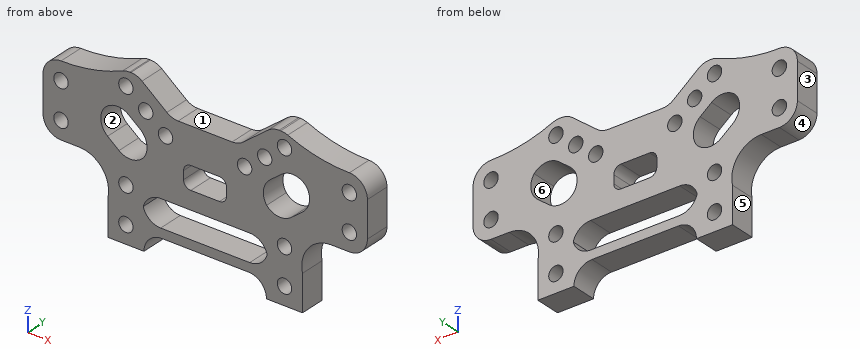
```python
from build123d import *

# Parameters (mm, degrees)
F0_R        = 1
F1_DEPTH    = 3.5
F2_R        = 2.49999
F3_W        = 8.6775156483
F3_H        = 3.7365088891
F4_DEPTH    = 25.4
F5_T1_DEPTH = 3.5
F6_W        = 5.9684215951
F6_H        = 3.1480632909
F7_DEPTH    = 25.4
F8_R        = 1


# Not quite as in the source:
# - a fillet or chamfer that OpenCascade refuses, or shapes differently, is made with other operations: its cross-section is extruded or revolved along the edge and cut away or added
# - a fillet or chamfer is up to 0.001 mm smaller than in the source, because OpenCascade refuses the exact size


with BuildPart() as f1:
    # F0 (on Front) → F1 (new body)
    with BuildSketch(Plane.XZ):
        with BuildLine():
            Line((-13.8224843517, 17.5), (-13.8224843517, 10))
            Line((-13.8224843517, 10), (-13.8224843517, 7.5))
            Line((-13.8224843517, 7.5), (-8.8224843517, 7.5))
            ThreePointArc((-8.8224843517, 7.5), (-5.620922233, 5.961249695), (-4.8224843517, 2.5))
            Line((-4.8224843517, 2.5), (-4.8224843517, 0))
            Line((-4.8224843517, 0), (-4.8224843517, -2.5))
            Line((-4.8224843517, -2.5), (0.1775156483, -2.5))
            Line((0.1775156483, -2.5), (0.1775156483, 0))
            Line((0.1775156483, 0), (8.6775156483, 0))
            Line((8.6775156483, 0), (17.1775156483, 0))
            Line((17.1775156483, 0), (17.1775156483, -2.5))
            Line((17.1775156483, -2.5), (22.1775156483, -2.5))
            Line((22.1775156483, -2.5), (22.1775156483, 0))
            Line((22.1775156483, 0), (22.1775156483, 2.5))
            ThreePointArc((22.1775156483, 2.5), (22.9759535296, 5.961249695), (26.1775156483, 7.5))
            Line((26.1775156483, 7.5), (31.1775156483, 7.5))
            Line((31.1775156483, 7.5), (31.1775156483, 10))
            Line((31.1775156483, 10), (31.1775156483, 17.5))
            Line((31.1775156483, 17.5), (28.6775156483, 17.5))
            ThreePointArc((28.6775156483, 17.5), (24.0740626287, 17.9907408644), (19.6775156483, 19.4409066995))
            Line((19.6775156483, 19.4409066995), (18.069904763, 19.4409066995))
            Line((18.069904763, 19.4409066995), (13.2764897522, 15.6480632909))
            Line((13.2764897522, 15.6480632909), (4.0469631395, 15.6480632909))
            Line((4.0469631395, 15.6480632909), (-0.7712156733, 19.4605013357))
            Line((-0.7712156733, 19.4605013357), (-2.3224843517, 19.4605013357))
            ThreePointArc((-2.3224843517, 19.4605013357), (-6.7169560029, 17.9958056322), (-11.3224843517, 17.5))
            Line((-11.3224843517, 17.5), (-13.8224843517, 17.5))
        make_face()
        with Locations((-2.3224843517, 0)):
            Circle(F0_R, mode=Mode.SUBTRACT)
        with Locations((-2.3224843517, 5)):
            Circle(F0_R, mode=Mode.SUBTRACT)
        with BuildLine():
            ThreePointArc((18.6775156483, 0), (19.6775156483, 1), (20.6775156483, 0))
            ThreePointArc((20.6775156483, 0), (19.6775156483, -1), (18.6775156483, 0))
        make_face(mode=Mode.SUBTRACT)
        with Locations((19.6775156483, 5)):
            Circle(F0_R, mode=Mode.SUBTRACT)
        with BuildLine():
            ThreePointArc((-12.3224843517, 10), (-11.3224843517, 11), (-10.3224843517, 10))
            ThreePointArc((-10.3224843517, 10), (-11.3224843517, 9), (-12.3224843517, 10))
        make_face(mode=Mode.SUBTRACT)
        with Locations((3.1775156483, 13.1480632909)):
            Circle(F0_R, mode=Mode.SUBTRACT)
        with Locations((-11.3224843517, 15)):
            Circle(F0_R, mode=Mode.SUBTRACT)
        with Locations((0.4275156483, 15.3240316454)):
            Circle(F0_R, mode=Mode.SUBTRACT)
        with Locations((-2.3224843517, 17.5)):
            Circle(F0_R, mode=Mode.SUBTRACT)
        with Locations((14.1459372434, 13.1480632909)):
            Circle(F0_R, mode=Mode.SUBTRACT)
        with Locations((28.6775156483, 10)):
            Circle(F0_R, mode=Mode.SUBTRACT)
        with Locations((16.9275156483, 15.3240316454)):
            Circle(F0_R, mode=Mode.SUBTRACT)
        with Locations((19.6775156483, 17.5)):
            Circle(F0_R, mode=Mode.SUBTRACT)
        with Locations((28.6775156483, 15)):
            Circle(F0_R, mode=Mode.SUBTRACT)
    extrude(amount=F1_DEPTH)

    # F2 (radius 2.5 in the source; OpenCascade refuses exactly that, so slightly less here)
    f2_edges = [f1.edges().sort_by_distance(p)[0] for p in [
        (-13.822484, -1.75, 17.5),
        (-13.822484, -1.75, 7.5),
        (31.177516, -1.75, 7.5),
        (31.177516, -1.75, 17.5),
        (-2.322484, -1.75, 19.460501),
        (-0.771216, -1.75, 19.460501),
        (4.046963, -1.75, 15.648063),
        (13.27649, -1.75, 15.648063),
        (18.069905, -1.75, 19.440907),
        (19.677516, -1.75, 19.440907),
        (0.177516, -1.75, 0),
        (17.177516, -1.75, 0),
    ]]
    fillet(f2_edges, radius=F2_R)

    # F3 (on face) → F4 (cut)
    with BuildSketch(Plane.XZ.offset(3.5)):
        Polygon((1.6262469699, 11.1875619551), (-3.8737530301, 15.5394986643), (-6.8168965969, 11.8199386845), (-1.3168965969, 7.4680019754), align=None)
        with Locations((4.3387578242, 3.1317455554)):
            Rectangle(F3_W, F3_H)
        with Locations((13.0162734725, 3.1317455554)):
            Rectangle(F3_W, F3_H)
        Polygon((24.1719278936, 11.8199386845), (21.2287843267, 15.5394986643), (15.7287843267, 11.1875619551), (18.6719278936, 7.4680019754), align=None)
    extrude(amount=-F4_DEPTH, mode=Mode.SUBTRACT)

    # F5: fillet of radius 2.5 on 12 edges, made by hand

    # F5_s2 → F5_t1 (join)
    with BuildSketch(Plane.XZ):
        with BuildLine():
            ThreePointArc((-5.4250217085, 13.5789973285), (-3.7538915599, 14.5109250411), (-1.9132516944, 13.9882299859))
            Line((-1.9132516944, 13.9882299859), (-3.8737530301, 15.5394986643))
            Line((-3.8737530301, 15.5394986643), (-5.4250217085, 13.5789973285))
        make_face()
        with BuildLine():
            ThreePointArc((-5.2656279185, 13.7804400203), (-5.7883229738, 11.9398001548), (-4.8563952612, 10.2686700061))
            Line((-4.8563952612, 10.2686700061), (-6.8168965969, 11.8199386845))
            Line((-6.8168965969, 11.8199386845), (-5.2656279185, 13.7804400203))
        make_face()
        with BuildLine():
            ThreePointArc((-3.2773979327, 9.0192706538), (-1.4367580672, 8.4965755986), (0.2343720815, 9.4285033111))
            Line((0.2343720815, 9.4285033111), (-1.3168965969, 7.4680019754))
            Line((-1.3168965969, 7.4680019754), (-3.2773979327, 9.0192706538))
        make_face()
        with BuildLine():
            ThreePointArc((0.0749782915, 9.2270606194), (0.5976733467, 11.0677004849), (-0.3342543658, 12.7388306335))
            Line((-0.3342543658, 12.7388306335), (1.6262469699, 11.1875619551))
            Line((1.6262469699, 11.1875619551), (0.0749782915, 9.2270606194))
        make_face()
        with BuildLine():
            ThreePointArc((22.2114265578, 10.2686700061), (23.1433542704, 11.9398001548), (22.6206592151, 13.7804400203))
            Line((22.6206592151, 13.7804400203), (24.1719278936, 11.8199386845))
            Line((24.1719278936, 11.8199386845), (22.2114265578, 10.2686700061))
        make_face()
        with BuildLine():
            ThreePointArc((19.268282991, 13.9882299859), (21.1089228565, 14.5109250411), (22.7800530051, 13.5789973285))
            Line((22.7800530051, 13.5789973285), (21.2287843267, 15.5394986643))
            Line((21.2287843267, 15.5394986643), (19.268282991, 13.9882299859))
        make_face()
        with BuildLine():
            ThreePointArc((17.6892856624, 12.7388306335), (16.7573579499, 11.0677004849), (17.2800530051, 9.2270606194))
            Line((17.2800530051, 9.2270606194), (15.7287843267, 11.1875619551))
            Line((15.7287843267, 11.1875619551), (17.6892856624, 12.7388306335))
        make_face()
        with BuildLine():
            ThreePointArc((17.1206592151, 9.4285033111), (18.7917893638, 8.4965755986), (20.6324292293, 9.0192706538))
            Line((20.6324292293, 9.0192706538), (18.6719278936, 7.4680019754))
            Line((18.6719278936, 7.4680019754), (17.1206592151, 9.4285033111))
        make_face()
        with BuildLine():
            ThreePointArc((0, 3.7634911109), (0.732233047, 1.9957241579), (2.5, 1.2634911109))
            Line((2.5, 1.2634911109), (0, 1.2634911109))
            Line((0, 1.2634911109), (0, 3.7634911109))
        make_face()
        with BuildLine():
            ThreePointArc((0, 2.5), (0.732233047, 4.267766953), (2.5, 5))
            Line((2.5, 5), (0, 5))
            Line((0, 5), (0, 2.5))
        make_face()
        with BuildLine():
            ThreePointArc((17.3550312966, 2.5), (16.6227982496, 4.267766953), (14.8550312966, 5))
            Line((14.8550312966, 5), (17.3550312966, 5))
            Line((17.3550312966, 5), (17.3550312966, 2.5))
        make_face()
        with BuildLine():
            ThreePointArc((14.8550312966, 1.2634911109), (16.6227982496, 1.9957241579), (17.3550312966, 3.7634911109))
            Line((17.3550312966, 3.7634911109), (17.3550312966, 1.2634911109))
            Line((17.3550312966, 1.2634911109), (14.8550312966, 1.2634911109))
        make_face()
    extrude(amount=F5_T1_DEPTH)

    # F6 (on face) → F7 (cut)
    with BuildSketch(Plane.XZ.offset(3.5)):
        with Locations((8.6617264459, 9.0740316454)):
            Rectangle(F6_W, F6_H)
    extrude(amount=-F7_DEPTH, mode=Mode.SUBTRACT)

    # F8
    f8_edges = [f1.edges().sort_by_distance(p)[0] for p in [
        (5.677516, -1.75, 7.5),
        (5.677516, -1.75, 10.648063),
        (11.645937, -1.75, 7.5),
        (11.645937, -1.75, 10.648063),
    ]]
    fillet(f8_edges, radius=F8_R)


solid = f1.part
```
Check sheet for the modelled part. Datum: model origin and axes. Units: mm. Face numbers are marked on the shaded views. A direction names the side the tool comes from. Round coordinates to 2 decimals unless told otherwise and drop trailing zeros. Order: outer loops, then holes, each group sorted by start corner. A loop starts at its lowest first (then second) coordinate and runs counter-clockwise, first axis right, second up.
1) Scan lines: line 1 (Z direction, x = 3, y = -1.4); line 2 (Z direction, x = 2.5, y = -3.1); line 3 (X direction, y = -2.95, z = 13). Record each from-to range of solid material in increasing order.
2) Section check B-B (x = 25). Record the boundary of the cut face in (y, z).
3) Tool access check on the marked faces 1, 2 and 3. Record the directions out of +Z, -Z, +X, -X, +Y, -Y that give a thin tool (end or side, any length) a straight path to the whole face; none if there is none.
4) Mould release check, pull along Z, two halves, no side actions. Record for the marked faces 4, 5 and 6: +Z half, -Z half, draft (parallel to the pull), parting line (faces both ways), or undercut.
5) Section check A-A (y = -0.55). Give the number of separate pieces and of enclosed holes in the cut face, and give its area (3 significant figures).
6) Go/stop test with flat-tipped pins: pin 1 Ø1.6 at (x, z) = (16.93, 15.32) entering from -Y; pin 2 Ø1.8 at (x, y) = (10.5, -2) entering from +Z; pin 3 Ø1 at (x, y) = (10.5, -1) entering from -Z; pin 4 Ø2 at (x, y) = (27, -1) entering from -Z. Record where each tip stops, or that it passes through.
Result:
1. line 1: z = 0 to 1.26, 5 to 12.16, 14.13 to 16.48
1. line 2: z = -0.01 to 1.26, 5 to 12.41, 13.88 to 16.87
1. line 3: x = -13.82 to -5.68, -0.66 to 2.19, 4.17 to 13.16, 15.13 to 18.02, 23.04 to 31.18
2. outline: (-3.5, 7.33) - (0, 7.33) - (0, 17.81) - (-3.5, 17.81) - close
3. face 1: +Z, +Y, -Y
3. face 2: +Y, -Y
3. face 3: +Z, -Z, -X, +Y, -Y
4. face 4: -Z half
4. face 5: draft
4. face 6: undercut
5. separate pieces: 1
5. enclosed holes: 18
5. area: 505 mm2
6. pin 1: passes through
6. pin 2: stops at z = 15.65
6. pin 3: stops at z = 0
6. pin 4: stops at z = 7.5
